from build123d import *

# Parameters (mm, degrees)
SKETCH1_W                = 7
SKETCH1_H                = 4.4
SKETCH1_W_2              = 0.7
SKETCH1_H_2              = 0.7
SKETCH1_W_3              = 3.2
SKETCH1_H_3              = 1.5
BOSS_EXTRUDE1_DEPTH      = 4.25
SKETCH1_2_W              = 0.7
SKETCH1_2_H              = 0.7
BOSS_EXTRUDE2_DEPTH      = 1
BOSS_EXTRUDE3_START      = 4.25
SKETCH3_W                = 0.2
SKETCH3_H                = 0.4
BOSS_EXTRUDE3_DEPTH      = 3.25
LPATTERN1_COUNT          = 3
LPATTERN1_PITCH          = 1.25
BOSS_EXTRUDE4_DEPTH      = 0.8
BOSS_EXTRUDE4_DEPTH_BACK = 0.8


with BuildPart() as part:
    # Sketch1 → Boss-Extrude1 (new body)
    with BuildSketch(Plane.XY):
        Rectangle(SKETCH1_W, SKETCH1_H)
        Polygon((-2.5, 0.6), (-2.5, -1.7), (2.5, -1.7), (2.5, 0.6), (2, 0.6), (2, 0.1), (-2, 0.1), (-2, 0.6), align=None, mode=Mode.SUBTRACT)
        with Locations((-2.75, 1.45)):
            Rectangle(SKETCH1_W_2, SKETCH1_H_2, mode=Mode.SUBTRACT)
        with Locations((2.75, 1.45)):
            Rectangle(SKETCH1_W_2, SKETCH1_H_2, mode=Mode.SUBTRACT)
        with Locations((0, 1.05)):
            Rectangle(SKETCH1_W_3, SKETCH1_H_3, mode=Mode.SUBTRACT)
    extrude(amount=BOSS_EXTRUDE1_DEPTH)

    # Sketch1<2> → Boss-Extrude2 (add)
    with BuildSketch(Plane.XY):
        with Locations((2.75, 1.45)):
            Rectangle(SKETCH1_2_W, SKETCH1_2_H)
        Polygon((-2, 0.1), (-2, 0.6), (-2.5, 0.6), (-2.5, -1.7), (2.5, -1.7), (2.5, 0.6), (2, 0.6), (2, 0.1), align=None)
        with Locations((-2.75, 1.45)):
            Rectangle(SKETCH1_2_W, SKETCH1_2_H)
    extrude(amount=BOSS_EXTRUDE2_DEPTH)

    # Sketch3 → Boss-Extrude3 (add)
    with BuildSketch(Plane.XY.offset(BOSS_EXTRUDE3_START)):
        with Locations((1.05, -0.1)):
            Rectangle(SKETCH3_W, SKETCH3_H)
        with Locations((1.45, -0.1)):
            Rectangle(SKETCH3_W, SKETCH3_H)
    boss_extrude3 = extrude(amount=-BOSS_EXTRUDE3_DEPTH)

    # LPattern1: Boss-Extrude3 ×3
    with Locations(*[(-i * LPATTERN1_PITCH, 0, 0) for i in range(1, LPATTERN1_COUNT)]):
        add(boss_extrude3)

    # Sketch4 → Boss-Extrude4 (add, two sides)
    with BuildSketch(Plane(origin=(0, 0, 0), x_dir=(0, 0, -1), z_dir=(1, 0, 0))) as boss_extrude4_sk:
        Polygon((-2.125, 0.7), (-3.85, 0.3), (-2.125, 0.3), align=None)
    extrude(amount=BOSS_EXTRUDE4_DEPTH)
    extrude(boss_extrude4_sk.sketch, amount=-BOSS_EXTRUDE4_DEPTH_BACK)


solid = part.part
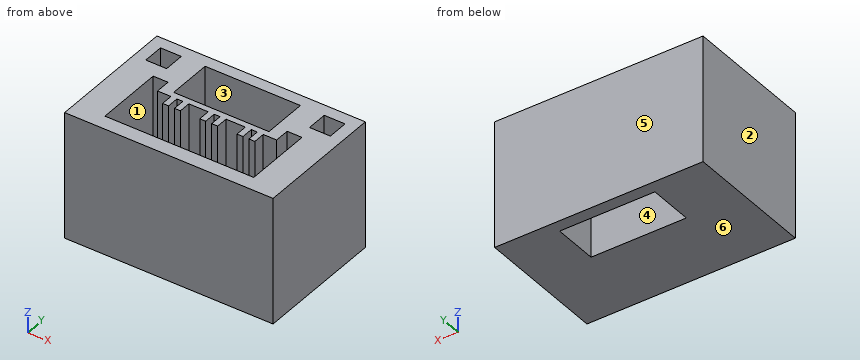
Source: CAD feature listing. Evaluate the final solid. Frame: model axes, mm. Face numbers are marked on the shaded views. A direction names the side the tool comes from. Coordinates: 2 decimals unless noted, no trailing zeros. Loops run counter-clockwise (first coordinate to the right, second up) from the corner with the lowest first, then second, coordinate; pieces in that order, holes last. Notation, with made-up numbers: (23.25, 12.25) - (73.25, 12.25) arc R24 ccw to (73.25, 24.25) - close; hole circle Ø3 at (32.25, -40). An arc over 180 degrees is marked (long way). One line per item, written item: value. Start each with the question number.
1. Contact query for a flat-ended pin moving along its axis: P1, Ø2, axis at x = 1.5, y = 1, coming from the +Z side. Output: stop coordinate, or through.
2. Section C-C (x = 1.25). Return the cut outline in (y, z), and give its area (4 significant figures).
3. Set-up query: the marked faces 1, 2 and 3. Return all of +Z, -Z, +X, -X, +Y, -Y with unobstructed straight access to the full face (end or side cutting, diameter ignored); none if empty.
4. Section A-A (y = 1.5). Return the cut outline in (x, z), and give its area (3 significant figures).
5. Section D-D (y = -1.05). Return the cut outline in (x, z).
6. Section B-B (x = -3). Return the cut outline in (y, z).
7. Ray query, L1, parallel to X at y = 1.5, z = 3.55; L2, parallel to Y at x = 0, z = 1.4; L3, parallel to Y at x = -1, z = 2.8. Return the intervals inside material, ascending.
8. Mould query, pull axis Y, two halves, no side actions, for the marked faces 4, 5 and 6. Classes: pulls with the +Y half, pulls with the -Y half, needs draft (parallel to the pull), parting line crosses it, or undercut.
Verdict:
1. P1: stops at z = 4.25
2. outline: (-2.2, 0) - (0.3, 0) - (0.3, 4.25) - (0.1, 4.25) - (0.1, 1) - (-1.7, 1) - (-1.7, 4.25) - (-2.2, 4.25) - close; (1.8, 0) - (2.2, 0) - (2.2, 4.25) - (1.8, 4.25) - close
2. area: 6.475 mm2
3. face 1: +Z
3. face 2: +Z, -Z, -X, +Y, -Y
3. face 3: +Z, -Z
4. outline: (-3.5, 0) - (-1.6, 0) - (-1.6, 4.25) - (-2.4, 4.25) - (-2.4, 1) - (-3.1, 1) - (-3.1, 4.25) - (-3.5, 4.25) - close; (1.6, 0) - (3.5, 0) - (3.5, 4.25) - (3.1, 4.25) - (3.1, 1) - (2.4, 1) - (2.4, 4.25) - (1.6, 4.25) - close
4. area: 11.6 mm2
5. outline: (-3.5, 0) - (3.5, 0) - (3.5, 4.25) - (2.5, 4.25) - (2.5, 1) - (-2.5, 1) - (-2.5, 4.25) - (-3.5, 4.25) - close
6. outline: (-2.2, 0) - (2.2, 0) - (2.2, 4.25) - (1.8, 4.25) - (1.8, 1) - (1.1, 1) - (1.1, 4.25) - (-2.2, 4.25) - close
7. L1: x = -3.5 to -3.1, -2.4 to -1.6, 1.6 to 2.4, 3.1 to 3.5
7. L2: y = -2.2 to -1.7, 0.1 to 0.3, 1.8 to 2.2
7. L3: y = -2.2 to -1.7, -0.3 to 0.3, 1.8 to 2.2
8. face 4: undercut
8. face 5: pulls with the +Y half
8. face 6: needs draft
